from build123d import *

# Parameters (mm, degrees)
SKETCH1_R               = 6
SKETCH1_R_2             = 3.05
BOSS_EXTRUDE1_DEPTH     = 7.5
SKETCH2_R               = 10.5
BOSS_EXTRUDE3_DEPTH     = 9
BOSS_EXTRUDE4_DEPTH     = 9
CIRPATTERN1_COUNT       = 14
SKETCH3_R               = 3.05
CUT_EXTRUDE1_DEPTH      = 10
SKETCH5_W               = 1.3
SKETCH5_H               = 8.98796618
BOSS_EXTRUDE5_DEPTH     = 16.5
SKETCH4_R               = 1.4
CUT_EXTRUDE2_DEPTH      = 1
CUT_EXTRUDE2_DEPTH_BACK = 38.540546983


with BuildPart() as part:
    # Sketch1 → Boss-Extrude1 (new body)
    with BuildSketch(Plane.XY):
        with Locations((-24.192657344, -27.82930415)):
            Circle(SKETCH1_R)
        with Locations((-24.192657344, -27.82930415)):
            Circle(SKETCH1_R_2, mode=Mode.SUBTRACT)
    extrude(amount=BOSS_EXTRUDE1_DEPTH)

    # Sketch2 → Boss-Extrude3 (add)
    with BuildSketch(Plane.XY.offset(7.5)):
        with Locations((-24.192657344, -27.82930415)):
            Circle(SKETCH2_R)
    extrude(amount=BOSS_EXTRUDE3_DEPTH)

    # Sketch2<4> → Boss-Extrude4 (add)
    with BuildSketch(Plane.XY.offset(7.5)):
        with BuildLine():
            ThreePointArc((-22.692657344, -17.436999304), (-22.822516009, -15.882132595), (-23.192657344, -14.366392132))
            ThreePointArc((-23.192657344, -14.366392132), (-24.192657344, -14.32930415), (-25.192657344, -14.366392132))
            ThreePointArc((-25.192657344, -14.366392132), (-25.562798679, -15.882132595), (-25.692657344, -17.436999304))
            ThreePointArc((-25.692657344, -17.436999304), (-24.192657344, -17.32930415), (-22.692657344, -17.436999304))
        make_face()
    boss_extrude4 = extrude(amount=BOSS_EXTRUDE4_DEPTH)

    # CirPattern1: Boss-Extrude4 ×14 about axis
    cirpattern1_axis = Axis((-24.192657344, -27.82930415, 0), (0, 0, 1))
    for i in range(1, CIRPATTERN1_COUNT):
        add(boss_extrude4.rotate(cirpattern1_axis, i * 360 / CIRPATTERN1_COUNT))

    # Sketch3 → Cut-Extrude1 (cut, through all)
    with BuildSketch(Plane(origin=(0, 0, 7.5), x_dir=(-1, 0, 0), z_dir=(0, 0, -1))):
        with Locations((24.192657344, -27.82930415)):
            Circle(SKETCH3_R)
    extrude(amount=-CUT_EXTRUDE1_DEPTH, mode=Mode.SUBTRACT)

    # Sketch5 → Boss-Extrude5 (add, through all)
    with BuildSketch(Plane(origin=(0, 0, 0), x_dir=(-1, 0, 0), z_dir=(0, 0, -1))):
        with Locations((21.792657344, -27.156324883)):
            Rectangle(SKETCH5_W, SKETCH5_H)
    extrude(amount=-BOSS_EXTRUDE5_DEPTH)

    # Sketch4 → Cut-Extrude2 (cut, two sides)
    with BuildSketch(Plane(origin=(0, 0, 0), x_dir=(0, 0, -1), z_dir=(1, 0, 0))) as cut_extrude2_sk:
        with Locations((-3.5, -27.82930415)):
            Circle(SKETCH4_R)
    extrude(amount=CUT_EXTRUDE2_DEPTH, mode=Mode.SUBTRACT)
    extrude(cut_extrude2_sk.sketch, amount=-CUT_EXTRUDE2_DEPTH_BACK, mode=Mode.SUBTRACT)


solid = part.part
Geometry: final body of the model. Coordinates: model frame, mm. A direction names the side the tool comes from. Coordinates: 2 decimals unless noted, no trailing zeros. Order: outer loops, then holes, each group sorted by start corner. A loop starts at its lowest first (then second) coordinate and runs counter-clockwise, first axis right, second up. Notation, with made-up numbers: M 49.5,63 L 59.5,63 A17 ccw 59.5,92 Z; hole C 75,88.25 d4. An arc over 180 degrees is marked long. One line per question, with ' | ' between items. Start each with the question number.
Item 1: Draft query along X for faces 5 (the cylindrical face through (-36.12, -29.14, 11.94)), 6 (the cylindrical face through (-24.21, -41.33, 11.94)), 7 (the cylindrical face through (-11.028, -24.839, 11.937)), 8 (the cylindrical face through (-26.52, -17.59, 11.94)). Return one class per face: released by +X, released by -X, zero draft, split by the parting line, or undercut.
Item 2: Cut plane B-B, the plane z = 1.25. Return the cut outline in (x, y).
Item 3: Pin query (flat end, axial travel): pin 1 Ø2 at (x, z) = (-33.5, 5) entering from +Y; pin 2 Ø3 at (y, z) = (-32.5, 9.5) entering from +X; pin 3 Ø5 at (x, z) = (-32.5, 5.5) entering from -Y; pin 4 Ø1.5 at (x, z) = (-27, 14) entering from -Y. Return the tip coordinate at first contact, or that it passes through.
Item 4: Set-up query: faces 1 (the cylindrical face through (-34.37, -34.19, 11.94)), 2 (the cylindrical face through (-35.514, -23.836, 11.937)), 3 (the cylindrical face through (-25.56, -15.86, 11.94)), 4 (the cylindrical face through (-12.22, -29.16, 11.94)). Return all of +Z, -Z, +X, -X, +Y, -Y with unobstructed straight access to the full face (end or side cutting, diameter ignored); none if empty.
Item 5: Cut plane A-A, the plane z = 3.5. Return the cut outline in (x, y), then the cut area to 3 significant figures.
Item 6: Ray query, probe 1 along X at (y, z) = (-40, 8); probe 2 along Y at (x, z) = (-30.25, 13.5); probe 3 along Z at (x, y) = (-15.25, -28.5). Return the intervals inside material, ascending. Write a range as [from, to].
A:
1) face 5: released by -X | face 6: split by the parting line | face 7: released by +X | face 8: undercut
2) outline: C -24.19,-27.83 d12; hole M -22.44,-30.33 L -22.44,-25.33 A3.05 ccw long Z
3) pin 1: passes through | pin 2: stops at x = -11.07 | pin 3: stops at y = -36.97 | pin 4: stops at y = -38.58
4) face 1: +Z, -Z, -X | face 2: +Z, -Z | face 3: +Z, -Z, +Y | face 4: +Z, -Z, +X
5) outline: M -30.03,-29.23 A6 ccw -18.36,-29.23 L -22.44,-29.23 L -22.44,-30.33 A3.05 cw -26.9,-29.23 Z; M -30.03,-26.43 L -26.9,-26.43 A3.05 cw -22.44,-25.33 L -22.44,-26.43 L -18.36,-26.43 A6 ccw Z | area: 68.3 mm2
6) probe 1: x = [-30.03, -28.77], [-25.52, -22.86], [-19.61, -18.35] | probe 2: y = [-39.89, -36.98], [-36.41, -19.25], [-18.68, -15.76] | probe 3: z = [7.5, 16.5]
